from build123d import *

# Parameters (mm, degrees)
SKETCH1_R           = 11
BOSS_EXTRUDE1_DEPTH = 35
FILLET2_R           = 25
FILLET5_R           = 5
CUT_EXTRUDE2_DEPTH  = 35
FILLET6_R           = 4
CUT_EXTRUDE1_DEPTH  = 20


with BuildPart() as part:
    # Sketch1 → Boss-Extrude1 (new body)
    with BuildSketch(Plane.XY):
        with BuildLine():
            Line((-47.101242547, -32.98064509), (-15.03971276, -10.530920247))
            ThreePointArc((-15.03971276, -10.530920247), (-11.176920202, -14.566045997), (-6.279523746, -17.252849698))
            Line((-6.279523746, -17.252849698), (31.308181085, -30.933655431))
            Line((31.308181085, -30.933655431), (43.278886102, 1.955586297))
            Line((43.278886102, 1.955586297), (12.982550619, 12.982550619))
            Line((12.982550619, 12.982550619), (40.658639918, 40.658639918))
            ThreePointArc((40.658639918, 40.658639918), (-36.960287557, 44.047555479), (-47.101242547, -32.98064509))
        make_face()
        Circle(SKETCH1_R, mode=Mode.SUBTRACT)
    extrude(amount=BOSS_EXTRUDE1_DEPTH)

    # Fillet2
    fillet2_edges = [part.edges().sort_by_distance(p)[0] for p in [
        (-15.03971276, -10.530920247, 17.5),
    ]]
    fillet(fillet2_edges, radius=FILLET2_R)

    # Fillet5
    fillet5_edges = [part.edges().sort_by_distance(p)[0] for p in [
        (12.982550619, 12.982550619, 17.5),
    ]]
    fillet(fillet5_edges, radius=FILLET5_R)

    # Sketch4 → Cut-Extrude2 (cut)
    with BuildSketch(Plane.XY.offset(35)):
        with BuildLine():
            Line((-41.656871027, -3.532188748), (-33.053224482, -15.819469412))
            Line((-33.053224482, -15.819469412), (-32.46214687, -15.405592412))
            ThreePointArc((-32.46214687, -15.405592412), (-23.62229066, -11.116679876), (-13.884259621, -9.809553241))
            ThreePointArc((-13.884259621, -9.809553241), (-16.986342471, 0.681299827), (-13.054027301, 10.890012453))
            Line((-13.054027301, 10.890012453), (-35.345481592, 37.455933189))
            ThreePointArc((-35.345481592, 37.455933189), (-49.017443505, 15.796842477), (-50.564853617, -9.769625307))
            Line((-50.564853617, -9.769625307), (-41.656871027, -3.532188748))
        make_face()
        with BuildLine():
            ThreePointArc((31.925370041, 40.410651415), (0.741106983, 51.494667301), (-30.749214933, 41.312658847))
            Line((-30.749214933, 41.312658847), (-8.457760642, 14.746738111))
            ThreePointArc((-8.457760642, 14.746738111), (1.75926732, 16.908724922), (11.312388901, 12.68975403))
            ThreePointArc((11.312388901, 12.68975403), (11.517857333, 18.111100205), (14.289586512, 22.774867886))
            Line((14.289586512, 22.774867886), (31.925370041, 40.410651415))
        make_face()
    extrude(amount=-CUT_EXTRUDE2_DEPTH, mode=Mode.SUBTRACT)

    # Fillet6
    fillet6_edges = [part.edges().sort_by_distance(p)[0] for p in [
        (-13.884259621, -9.809553241, 17.5),
        (-13.054027301, 10.890012453, 17.5),
        (-35.345481592, 37.455933189, 17.5),
        (-30.749214933, 41.312658847, 17.5),
        (-8.457760642, 14.746738111, 17.5),
        (11.312388901, 12.68975403, 17.5),
        (-50.564853617, -9.769625307, 17.5),
        (-33.053224482, -15.819469412, 17.5),
        (-41.656871027, -3.532188748, 17.5),
    ]]
    fillet(fillet6_edges, radius=FILLET6_R)

    # Sketch2 → Cut-Extrude1 (cut)
    with BuildSketch(Plane(origin=(37.587704831, -13.680805733, 0), x_dir=(0, 0, -1), z_dir=(0.939692620785907, -0.34202014332567265, 0))):
        with BuildLine():
            ThreePointArc((-6, -0.86009916), (-13.099140528, 9.764515464), (-25.631727984, 7.271628823))
            Line((-25.631727984, 7.271628823), (-9.368272016, -8.991827144))
            ThreePointArc((-9.368272016, -8.991827144), (-6.875385376, -5.260958632), (-6, -0.86009916))
        make_face()
        with BuildLine():
            Line((-9.368272016, -8.991827144), (-25.631727984, 7.271628823))
            ThreePointArc((-25.631727984, 7.271628823), (-25.631727984, -8.991827144), (-9.368272016, -8.991827144))
        make_face()
    extrude(amount=-CUT_EXTRUDE1_DEPTH, mode=Mode.SUBTRACT)


solid = part.part
Verification items for the finished model (mm, model axes). A direction names the side the tool comes from. Coordinates: 2 decimals unless noted, no trailing zeros. Write each loop counter-clockwise with the first axis right and the second up, starting at its lowest first coordinate (ties: lowest second). Pieces come first, ordered by that corner, then holes. Notation, with made-up numbers: (-32, 78) - (-4, 78) arc R7 cw to (-4, 84) - close; hole circle Ø3 at (-29.5, 50). An arc over 180 degrees is marked (long way). Answer as a JSON object with one key per item and string values.
(1) Gauge pin test, flat ends, axial feed: pin 1 Ø1.5 at (x, z) = (5, 8.5) entering from -Y; pin 2 Ø12 at (y, z) = (12.5, 12) entering from -X; pin 3 Ø1 at (x, z) = (-46.5, 14) entering from +Y. Record the tip position at first contact, or that the pin passes through.
Report:
{"pin 1": "y = -21.63", "pin 2": "x = -57.13", "pin 3": "y = 34.5"}
(2) Tool access check on faces 1 (the flat face through (29, 29, 17)), 2 (the flat face through (-19.287, 27.652, 17.745)), 3 (the flat face through (-38.19, -26.74, 17.26)). Record the directions out of +Z, -Z, +X, -X, +Y, -Y that give a thin tool (end or side, any length) a straight path to the whole face; none if there is none.
Report:
{"face 1": "+Z, -Z, +X", "face 2": "+Z, -Z", "face 3": "+Z, -Z, -Y"}
(3) Cross-section at A-A on x = 0. Record the cut outline in (y, z).
Report:
{"outline": "(-19.54, 0) - (-11, 0) - (-11, 35) - (-19.54, 35) - close; (11, 0) - (17, 0) - (17, 35) - (11, 35) - close; (51.5, 0) - (57.5, 0) - (57.5, 35) - (51.5, 35) - close"}
(4) Cross-section at B-B on x = 13. Record the cut outline in (y, z).
Report:
{"outline": "(-24.27, 0) - (21.22, 0) - (21.22, 35) - (-24.27, 35) - close; (49.83, 0) - (56.01, 0) - (56.01, 35) - (49.83, 35) - close"}
(5) Thickness scan on line 1 along Y through (x, z) = (-22, 31.5); line 2 along Y through (x, z) = (7, 7); line 3 along Y through (x, z) = (29, 16). Record the ranges inside material, lowest first.
Report:
{"line 1": "-16.89 to -10.68, 21.55 to 30.89, 46.56 to 53.12", "line 2": "-22.09 to -8.49, 8.49 to 15.59, 51.02 to 57.07", "line 3": "-30.09 to -23.6, 0.66 to 7.15, 29 to 37.49, 42.56 to 49.65"}
(6) Cross-section at C-C on z = 21.5. Give the number of separate pieces and of enclosed holes in the cut face, plus the area to 3 significant figures.
Report:
{"separate pieces": "1", "enclosed holes": "3", "area": "2,890 mm^2"}
(7) Mould release check, pull along Y, two halves, no side actions. Record for faces 4 (the cylindrical face through (-36.038, 44.806, 17.255)), 5 (the cylindrical face through (-16.897, 1.872, 17.745)), 6 (the flat face through (12.327, -24.025, 17.255)): pulls with the +Y half, pulls with the -Y half, needs draft (parallel to the pull), parting line crosses it, or undercut.
Report:
{"face 4": "parting line crosses it", "face 5": "undercut", "face 6": "pulls with the -Y half"}
